from build123d import *

# Parameters (mm, degrees)
F0_W      = 40
F0_H      = 40
F0_W_2    = 36
F0_H_2    = 36
F1_DEPTH  = 300
F2_R      = 16
F2_R_2    = 10
F3_DEPTH  = 25
F4_R      = 16
F4_R_2    = 4.25
F5_DEPTH  = 25
F6_R      = 10
F7_DEPTH  = 25
F8_R      = 4.25
F9_DEPTH  = 25
F10_R     = 2
F11_DEPTH = 25


with BuildPart() as f1:
    # F0 (on Front) → F1 (new body)
    with BuildSketch(Plane.XZ):
        with Locations((20, 20)):
            Rectangle(F0_W, F0_H)
        with Locations((20, 20)):
            Rectangle(F0_W_2, F0_H_2, mode=Mode.SUBTRACT)
    extrude(amount=F1_DEPTH)

    # F2 (on face) → F3 (cut)
    with BuildSketch(Plane.YZ.offset(40)):
        with Locations((-150, 20)):
            Circle(F2_R)
        with Locations((-190, 20)):
            Circle(F2_R_2)
        with Locations((-110, 20)):
            Circle(F2_R_2)
    extrude(amount=-F3_DEPTH, mode=Mode.SUBTRACT)

    # F4 (on face) → F5 (cut)
    with BuildSketch(Plane.YZ.offset(2)):
        with Locations((-150, 20)):
            Circle(F4_R)
        with Locations((-190, 20)):
            Circle(F4_R_2)
        with Locations((-110, 20)):
            Circle(F4_R_2)
    extrude(amount=-F5_DEPTH, mode=Mode.SUBTRACT)

    # F6 (on face) → F7 (cut)
    with BuildSketch(Plane.XY.offset(40)):
        with Locations((20, -280)):
            Circle(F6_R)
        with Locations((20, -20)):
            Circle(F6_R)
    extrude(amount=-F7_DEPTH, mode=Mode.SUBTRACT)

    # F8 (on face) → F9 (cut)
    with BuildSketch(Plane.XY.offset(2)):
        with Locations((20, -280)):
            Circle(F8_R)
        with Locations((20, -20)):
            Circle(F8_R)
    extrude(amount=-F9_DEPTH, mode=Mode.SUBTRACT)

    # F10 (on face) → F11 (cut)
    with BuildSketch(Plane(origin=(0, 0, 0), x_dir=(0, -1, 0), z_dir=(-1, 0, 0))):
        with Locations((128, 20)):
            Circle(F10_R)
        with Locations((172, 20)):
            Circle(F10_R)
    extrude(amount=-F11_DEPTH, mode=Mode.SUBTRACT)


solid = f1.part
Input: part model. Units: mm. Frame: model coordinates. A direction names the side the tool comes from. Round coordinates to 2 decimals unless told otherwise and drop trailing zeros. Loops run counter-clockwise (first coordinate to the right, second up) from the corner with the lowest first, then second, coordinate; pieces in that order, holes last. Notation, with made-up numbers: (-20.75, 74) -> (28.25, 74) arc R34 ccw to (28.25, 106) -> close; hole circle Ø9 at (25.25, 36). An arc over 180 degrees is marked (long way). Answer as a JSON object with one key per item and string values. Group by question number.
1) Ray query, L1, parallel to Y at x = 20, z = 38.85; L2, parallel to X at y = -132, z = 17. Return the intervals inside material, ascending.
2) Reachability of faces 1 (the cylindrical face through (29.54, -17, 39.01)), 2 (the flat face through (20, -148, 38)), 3 (the flat face through (18, 0, 1)), 4 (the cylindrical face through (39.014, -180.763, 16.17)) from +Z, -Z, +X, -X, +Y, -Y: full face, straight path, thin tool, end or side. Return the list, or none.
3) Pin query (flat end, axial travel): pin 1 (18 mm diameter, centred on x = 20, y = -280, fed in from +Z); pin 2 (5 mm diameter, centred on y = -104, z = 5, fed in from -X); pin 3 (7 mm diameter, centred on x = 20, y = -20, fed in from +Z); pin 4 (13.5 mm diameter, centred on y = -110, z = 20, fed in from +X). Return the tip coordinate at first contact, or that it passes through.
4) Section query B-B on y = -65. Output: boundary loops of the cut face in (x, z), plus the area to 3 significant figures.
5) Section query A-A on y = -110. Output: boundary loops of the cut face in (x, z), plus the area to 3 significant figures.
6) Section query C-C on y = -150. Output: boundary loops of the cut face in (x, z).
7) Draft query along X for faces 5 (the flat face through (40, -148, 2)), 6 (the cylindrical face through (39.014, -162.697, 10.264)), 7 (the cylindrical face through (19.447, -275.786, 1.014)). Return one class per face: +X half, -X half, draft (parallel to the pull), parting line (faces both ways), or undercut.
Reply:
{
 "1": {"L1": "y = -300 to -290, -270 to -30, -10 to 0", "L2": "x = 0 to 2, 38 to 40"},
 "2": {"face 1": "+Z", "face 2": "+Y, -Y", "face 3": "+Z, -Z, +X, -X, +Y", "face 4": "+X"},
 "3": {"pin 1": "stops at z = 2", "pin 2": "stops at x = 0", "pin 3": "passes through", "pin 4": "stops at x = 2"},
 "4": {"outline": "(0, 0) -> (40, 0) -> (40, 40) -> (0, 40) -> close; hole (2, 2) -> (38, 2) -> (38, 38) -> (2, 38) -> close", "area": "304 mm2"},
 "5": {"outline": "(0, 0) -> (40, 0) -> (40, 10) -> (38, 10) -> (38, 2) -> (2, 2) -> (2, 15.75) -> (0, 15.75) -> close; (0, 24.25) -> (2, 24.25) -> (2, 38) -> (38, 38) -> (38, 30) -> (40, 30) -> (40, 40) -> (0, 40) -> close", "area": "247 mm2"},
 "6": {"outline": "(0, 0) -> (40, 0) -> (40, 4) -> (38, 4) -> (38, 2) -> (2, 2) -> (2, 4) -> (0, 4) -> close; (0, 36) -> (2, 36) -> (2, 38) -> (38, 38) -> (38, 36) -> (40, 36) -> (40, 40) -> (0, 40) -> close"},
 "7": {"face 5": "+X half", "face 6": "draft", "face 7": "undercut"}
}
